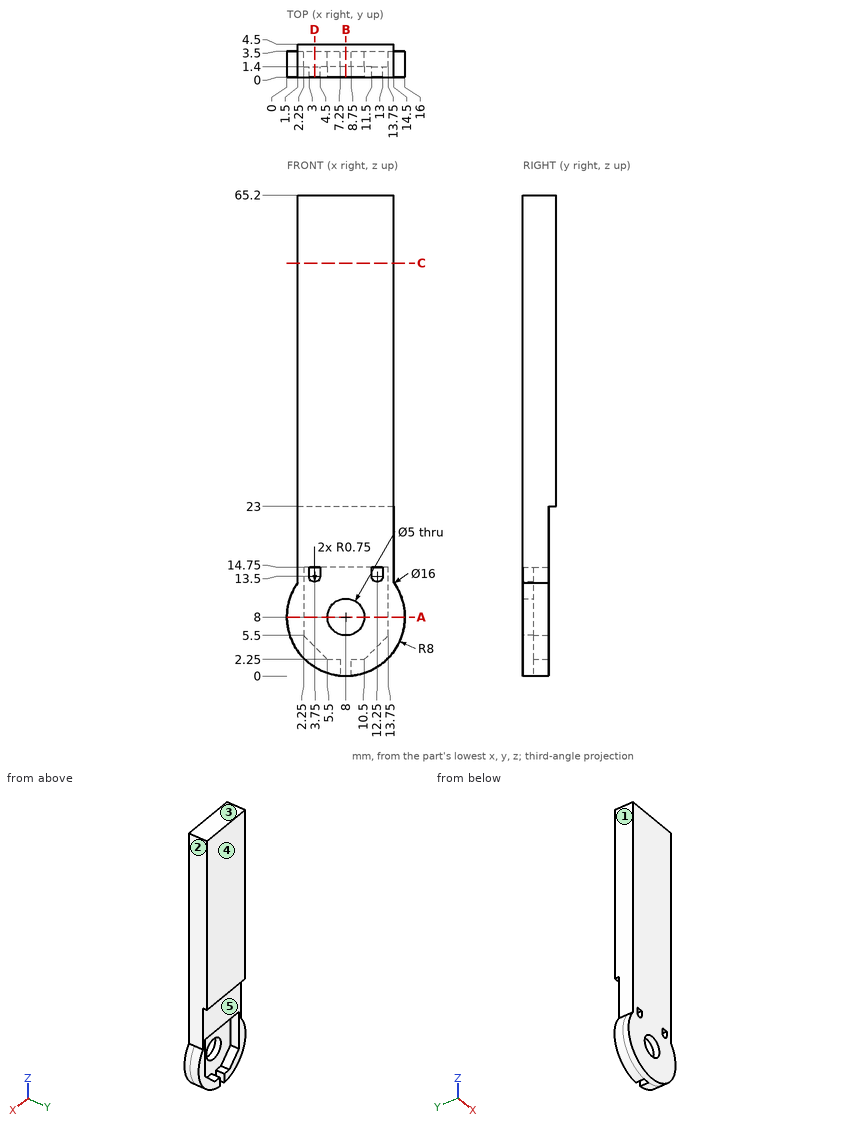
For this review, use the dimensioned drawing (mm, ordinates from the lowest corner) and the shaded views. A direction names the side the tool comes from. Round coordinates to 2 decimals unless told otherwise and drop trailing zeros. Order: outer loops, then holes, each group sorted by start corner. A loop starts at its lowest first (then second) coordinate and runs counter-clockwise, first axis right, second up. Notation, with made-up numbers: M 72,35.5 L 83,35.5 A15 cw 83,54.5 Z; hole C 19,45.5 d1. An arc over 180 degrees is marked long. Write each question's results on one line, items separated by ' | '. Start each with the question number.
1. Add section D-D (x = 3.75). State the section outline as (y, z) points.
2. Clearance check with flat-ended pins moving along their axes: pin 1 Ø0.6 at (y, z) = (0.5, 14) entering from +X; pin 2 Ø1 at (x, y) = (9, 2.5) entering from -Z; pin 3 Ø2 at (x, y) = (11.5, 0.5) entering from -Z. State where each tip first meets the part, or that it passes through.
3. Tool access review of the marked faces 1, 2, 3, 4 and 5: name each direction out of +Z, -Z, +X, -X, +Y, -Y from which nothing blocks a thin tool from reaching the whole face with its end or side.
4. To check wall thickness, follow L1, parallel to X at y = 1.05, z = 8; L2, parallel to Y at x = 4.5, z = 13; L3, parallel to X at y = 1.8, z = 43.5. State the ranges of each line that lie inside material, in increasing order. Write a range as [from, to].
5. Add section A-A (z = 8). State the section outline as (x, y) points, then the cut area to 4 significant figures.
6. Add section C-C (z = 56). State the section outline as (x, y) points.
7. Add section B-B (x = 8). State the section outline as (y, z) points.
Output values:
1) outline: M 0,1.22 L 3.5,1.22 L 3.5,4 L 1.4,4 L 1.4,12.75 L 0,12.75 Z; M 0,14.75 L 3.5,14.75 L 3.5,23 L 4.5,23 L 4.5,65.2 L 0,65.2 Z
2) pin 1: x = 14.5 | pin 2: z = 0.04 | pin 3: z = 0.4
3) face 1: +Z, -X, +Y, -Y | face 2: +Z, +X, +Y, -Y | face 3: +Z, +X, -X, +Y, -Y | face 4: +Z, -Z, +X, -X, +Y | face 5: -Z, +X, -X, +Y
4) L1: [0, 5.5], [10.5, 16] | L2: [0, 1.4] | L3: [1.5, 14.5]
5) outline: M 0,0 L 5.5,0 L 5.5,1.4 L 2.25,1.4 L 2.25,3.5 L 0,3.5 Z; M 10.5,0 L 16,0 L 16,3.5 L 13.75,3.5 L 13.75,1.4 L 10.5,1.4 Z | area: 24.85 mm^2
6) outline: M 1.5,0 L 14.5,0 L 14.5,4.5 L 1.5,4.5 Z
7) outline: M 0,0 L 1.4,0 L 1.4,5.5 L 0,5.5 Z; M 0,10.5 L 1.4,10.5 L 1.4,14.75 L 3.5,14.75 L 3.5,23 L 4.5,23 L 4.5,65.2 L 0,65.2 Z
